from build123d import *

# Parameters (mm, degrees)
SKETCH_1_W               = 59
SKETCH_1_H               = 100
EXTRUDE_1_DEPTH          = 24
SKETCH_3_R               = 1.45
SKETCH_3_R_2             = 1.7
CUT_EXTRUDE_1_DEPTH      = 85.1546196
CUT_EXTRUDE_2_DEPTH      = 67.867406111
SKETCH_5_W               = 42
SKETCH_5_H               = 59
SKETCH_5_R               = 1.6
EXTRUDE_2_DEPTH          = 2
EXTRUDE_3_DEPTH          = 1.5
CUT_EXTRUDE_3_DEPTH      = 91.709701842
CUT_EXTRUDE_3_DEPTH_BACK = 91.709701842
SKETCH_9_R               = 1.5
CUT_EXTRUDE_4_DEPTH      = 115.002192998


with BuildPart() as part:
    # 草图1 → 凸台-拉伸1 (new body)
    with BuildSketch(Plane.XY):
        with Locations((0, -5)):
            Rectangle(SKETCH_1_W, SKETCH_1_H)
    extrude(amount=EXTRUDE_1_DEPTH)

    # 草图3 → 切除-拉伸1 (cut, through all)
    with BuildSketch(Plane.ZY.offset(29.5)):
        with Locations(Location((12, -38, 0), (0, 0, 270))):
            Circle(SKETCH_3_R)
        with Locations(Location((12, -45, 0), (0, 0, 270))):
            Circle(SKETCH_3_R_2)
        with Locations(Location((19, -45, 0), (0, 0, 270))):
            Circle(SKETCH_3_R)
        with Locations(Location((12, -52, 0), (0, 0, 270))):
            Circle(SKETCH_3_R)
        with Locations(Location((5, -45, 0), (0, 0, 270))):
            Circle(SKETCH_3_R)
    extrude(amount=-CUT_EXTRUDE_1_DEPTH, mode=Mode.SUBTRACT)

    # 草图4 → 切除-拉伸2 (cut, through all)
    with BuildSketch(Plane.XY.offset(24)):
        Polygon((-24.5, -13.483129661), (-24.5, -30.715572957), (-26.5, -30.715572957), (-26.5, -55), (26.5, -55), (26.5, -30.715572957), (24.5, -30.715572957), (24.5, -13.483129661), align=None)
        Polygon((-29.5, 45), (-29.5, -10.991548546), (-24.5, 1.098015798), (-18.873933883, 45), align=None)
        Polygon((24.5, 1.098015798), (29.5, -10.991548546), (29.5, 45), (18.873933883, 45), align=None)
        Polygon((-1.5, 43.003983046), (-16, 43.003983046), (-21, 1.098015798), (-21, -10.656485647), (-1.5, -10.656485647), align=None)
        Polygon((21, 1.098015798), (16, 43.003983046), (1.5, 43.003983046), (1.5, -10.656485647), (21, -10.656485647), align=None)
    extrude(amount=-CUT_EXTRUDE_2_DEPTH, mode=Mode.SUBTRACT)

    # 草图5 → 凸台-拉伸2 (add, symmetric)
    with BuildSketch(Plane(origin=(0, 45, 0), x_dir=(1, 0, 0), z_dir=(0, 1, 0))):
        with Locations((0, -12)):
            Rectangle(SKETCH_5_W, SKETCH_5_H)
        with Locations(Location((-17, 15, 0), (0, 0, 270))):
            Circle(SKETCH_5_R, mode=Mode.SUBTRACT)
        with Locations(Location((-12.737493843, 8.230137279, 0), (0, 0, 270))):
            Circle(SKETCH_5_R, mode=Mode.SUBTRACT)
        with Locations(Location((12.737493843, 8.230137279, 0), (0, 0, 270))):
            Circle(SKETCH_5_R, mode=Mode.SUBTRACT)
        with Locations(Location((17, 15, 0), (0, 0, 270))):
            Circle(SKETCH_5_R, mode=Mode.SUBTRACT)
        with Locations(Location((17, -39, 0), (0, 0, 270))):
            Circle(SKETCH_5_R, mode=Mode.SUBTRACT)
        with Locations(Location((12.737493843, -32.230137279, 0), (0, 0, 270))):
            Circle(SKETCH_5_R, mode=Mode.SUBTRACT)
        with Locations(Location((-17, -39, 0), (0, 0, 270))):
            Circle(SKETCH_5_R, mode=Mode.SUBTRACT)
        with Locations(Location((-12.737493843, -32.230137279, 0), (0, 0, 270))):
            Circle(SKETCH_5_R, mode=Mode.SUBTRACT)
    extrude(amount=EXTRUDE_2_DEPTH, both=True)

    # 草图7 → 凸台-拉伸3 (add, symmetric)
    with BuildSketch(Plane(origin=(0, 0, 0), x_dir=(0, 0, 1), z_dir=(1, 0, 0))):
        with BuildLine():
            Line((0, -43), (0, 11.218667819))
            Line((0, 11.218667819), (-1.377914125, 1.87990225))
            add(Edge.make_bspline(
                [(-17.5, -43), (-6.662948015, -38.990116627), (-2.969302536, -28.650335037), (-2.475614958, -10.791960979), (-1.377914125, 1.87990225)],
                knots=[0, 0, 0, 0, 0, 1, 1, 1, 1, 1], degree=4))
            Line((-17.5, -43), (0, -43))
        make_face()
        with BuildLine():
            Line((24, -43), (41.5, -43))
            add(Edge.make_bspline(
                [(41.5, -43), (30.662948015, -38.990116627), (26.969302536, -28.650335037), (26.475614958, -10.791960979), (25.377914125, 1.87990225)],
                knots=[0, 0, 0, 0, 0, 1, 1, 1, 1, 1], degree=4))
            Line((25.377914125, 1.87990225), (24, 11.218667819))
            Line((24, 11.218667819), (24, -43))
        make_face()
    extrude(amount=EXTRUDE_3_DEPTH, both=True)

    # 草图8 → 切除-拉伸3 (cut, two sides: drawn at the far end of the back side and taken through both)
    with BuildSketch(Plane(origin=(29.5, 0, 0), x_dir=(0, 0, -1), z_dir=(1, 0, 0)).offset(-CUT_EXTRUDE_3_DEPTH_BACK)):
        with BuildLine():
            Line((-24, -55), (-12, -55))
            ThreePointArc((-12, -55), (-19.810249676, -52.172299611), (-24, -45))
            Line((-24, -45), (-24, -55))
        make_face()
        with BuildLine():
            Line((0, -55), (0, -45))
            ThreePointArc((0, -45), (-4.189750324, -52.172299611), (-12, -55))
            Line((-12, -55), (0, -55))
        make_face()
    extrude(amount=CUT_EXTRUDE_3_DEPTH + CUT_EXTRUDE_3_DEPTH_BACK, mode=Mode.SUBTRACT)

    # 草图9 → 切除-拉伸4 (cut, through all)
    with BuildSketch(Plane(origin=(0, 47, 0), x_dir=(1, 0, 0), z_dir=(0, 1, 0))):
        with Locations(Location((-7, -12, 0), (0, 0, 270))):
            Circle(SKETCH_9_R)
        with Locations(Location((7, -12, 0), (0, 0, 270))):
            Circle(SKETCH_9_R)
    extrude(amount=-CUT_EXTRUDE_4_DEPTH, mode=Mode.SUBTRACT)


solid = part.part
Design review of the part built by this model. Coordinates are the model's own, in mm. A direction names the side the tool comes from. Give positions to 0.01 mm unless a question says otherwise; leave off trailing zeros. Write each loop counter-clockwise with the first axis right and the second up, starting at its lowest first coordinate (ties: lowest second). Pieces come first, ordered by that corner, then holes. Notation, with made-up numbers: M 74,-5 L 108,-5 A6 ccw 108,-1 Z; hole C 61,31 d8. An arc over 180 degrees is marked long. Return JSON: item names as keys, results as strings. Group by question number.
Item 1: Take a section at B-B (y = -19). Give the boundary of the cut face in (x, z).
Item 2: Take a section at A-A (y = -42). Give the boundary of the cut face in (x, z), plus the area to 3 significant figures.
Item 3: Take a section at C-C (z = 5). Count the separate pieces of the cut face and the enclosed holes in it, plus the area to 3 significant figures.
Item 4: Clearance check with flat-ended pins moving along their axes: pin 1 Ø6 at (x, z) = (-7.5, 8.5) entering from -Y; pin 2 Ø1.5 at (x, y) = (20.5, 34) entering from +Z; pin 3 Ø4 at (x, z) = (17, 39) entering from -Y. State where each tip first meets the part, or that it passes through.
Item 5: Wall thickness on line 1 along Y through (x, z) = (-7, 16); line 2 along Z through (x, y) = (28.35, -45); line 3 along Z through (x, y) = (28, -38): over which ranges is each line inside the solid? List them lowest first.
Item 6: Tool access review of faces 4 (the cylindrical face through (18.586, 44.972, 38.792)), 5 (the flat face through (-21, -5, 12)), 6 (the flat face through (-29.5, -33, 12)), 7 (the flat face through (26.5, -43, 12)), 8 (the flat face through (-21.853, 21.756, 12.168)): name each direction out of +Z, -Z, +X, -X, +Y, -Y from which nothing blocks a thin tool from reaching the whole face with its end or side.
Item 7: The part is to be moulded in two halves that separate along X. For faces 1 (the flat face through (-0.02, -6.61, -0.68)), 2 (the flat face through (-11, -10.656, 12)), 3 (the flat face through (26.965, -4.862, 12.168)), say which applies: pulls with the +X half, pulls with the -X half, needs draft (parallel to the pull), parting line crosses it, or undercut.
Return value:
{
 "1": {"outline": "M -29.5,0 L -24.5,0 L -24.5,24 L -29.5,24 Z; M 24.5,0 L 29.5,0 L 29.5,24 L 24.5,24 Z"},
 "2": {"outline": "M -29.5,0 L -26.5,0 L -26.5,24 L -29.5,24 Z; M 26.5,0 L 29.5,0 L 29.5,24 L 26.5,24 Z", "area": "144 mm2"},
 "3": {"separate pieces": "3", "enclosed holes": "2", "area": "1,200 mm2"},
 "4": {"pin 1": "stops at y = -13.48", "pin 2": "stops at z = 24", "pin 3": "stops at y = 43"},
 "5": {"line 1": "y = -13.48 to -10.66, 43 to 47", "line 2": "z = 0 to 3.55, 6.45 to 10.3, 13.7 to 17.55, 20.45 to 24", "line 3": "z = 0 to 10.55, 13.45 to 24"},
 "6": {"face 4": "+Y, -Y", "face 5": "+Z, -Z", "face 6": "+Z, -Z, -X, +Y, -Y", "face 7": "+Z, -Z, -Y", "face 8": "+Z, -Z, -X"},
 "7": {"face 1": "needs draft", "face 2": "undercut", "face 3": "pulls with the +X half"}
}
